Verification items for the finished model (mm, model axes). Face numbers are marked on the shaded views. A direction names the side the tool comes from. Coordinates: 2 decimals unless noted, no trailing zeros. Write each loop counter-clockwise with the first axis right and the second up, starting at its lowest first coordinate (ties: lowest second). Pieces come first, ordered by that corner, then holes. Notation, with made-up numbers: M 20.25,8.25 L 42.25,8.25 A24 ccw 42.25,18.25 Z; hole C -22.5,-13.75 d3. An arc over 180 degrees is marked long. One line per item, written item: value.
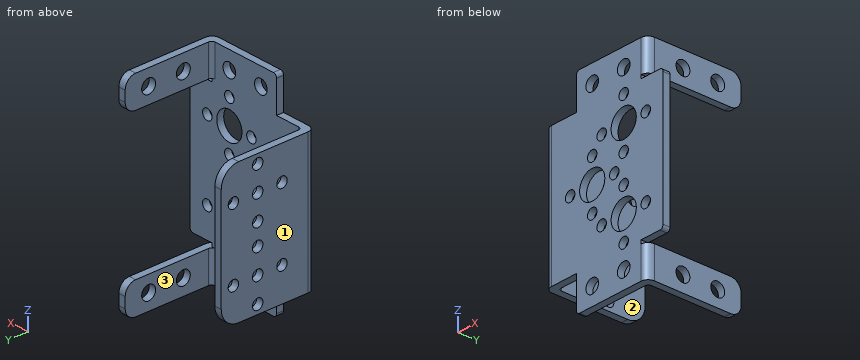
```python
from build123d import *

# Parameters (mm, degrees)
SKETCH1_W           = 35.49
SKETCH1_H           = 39
BOSS_EXTRUDE1_DEPTH = 2
SKETCH2_W           = 20.5
SKETCH2_H           = 10
BOSS_EXTRUDE2_DEPTH = 2
SKETCH3_W           = 39
SKETCH3_H           = 27
BOSS_EXTRUDE3_DEPTH = 2
SKETCH4_W           = 9
SKETCH4_H           = 27
BOSS_EXTRUDE4_DEPTH = 2
SKETCH5_R           = 4
SKETCH5_R_2         = 2
SKETCH5_R_3         = 1.5
CUT_EXTRUDE1_DEPTH  = 2
SKETCH6_R           = 2
CUT_EXTRUDE2_DEPTH  = 2
SKETCH7_R           = 1.5
CUT_EXTRUDE3_DEPTH  = 2
FILLET1_R           = 2
FILLET2_R           = 1
FILLET3_R           = 3
FILLET4_R           = 5


with BuildPart() as part:
    # Sketch1 → Boss-Extrude1 (new body)
    with BuildSketch(Plane(origin=(0, 0, 0), x_dir=(1, 0, 0), z_dir=(0, 1, 0))):
        Rectangle(SKETCH1_W, SKETCH1_H)
    extrude(amount=BOSS_EXTRUDE1_DEPTH)

    # Sketch2 → Boss-Extrude2 (add)
    with BuildSketch(Plane(origin=(0, 2, 0), x_dir=(1, 0, 0), z_dir=(0, 1, 0))):
        with Locations((0.505, 24.5)):
            Rectangle(SKETCH2_W, SKETCH2_H)
        with Locations((0.505, -24.5)):
            Rectangle(SKETCH2_W, SKETCH2_H)
    extrude(amount=-BOSS_EXTRUDE2_DEPTH)

    # Sketch3 → Boss-Extrude3 (add)
    with BuildSketch(Plane.ZY.offset(17.745)):
        with Locations((0, 13.5)):
            Rectangle(SKETCH3_W, SKETCH3_H)
    extrude(amount=BOSS_EXTRUDE3_DEPTH)

    # Sketch4 → Boss-Extrude4 (add)
    with BuildSketch(Plane(origin=(10.755, 0, 0), x_dir=(0, 0, -1), z_dir=(1, 0, 0))):
        with Locations((-25, 13.5)):
            Rectangle(SKETCH4_W, SKETCH4_H)
        with Locations((25, 13.5)):
            Rectangle(SKETCH4_W, SKETCH4_H)
    extrude(amount=BOSS_EXTRUDE4_DEPTH)

    # Sketch5 → Cut-Extrude1 (cut)
    with BuildSketch(Plane(origin=(0, 2, 0), x_dir=(1, 0, 0), z_dir=(0, 1, 0))):
        with Locations((-4.755, 0)):
            Circle(SKETCH5_R)
        with Locations((5.245, 11)):
            Circle(SKETCH5_R)
        with Locations((5.245, -11)):
            Circle(SKETCH5_R)
        with Locations((-4.755, -24.5)):
            Circle(SKETCH5_R_2)
        with Locations((5.245, -24.5)):
            Circle(SKETCH5_R_2)
        with Locations((5.245, 24.5)):
            Circle(SKETCH5_R_2)
        with Locations((5.245, 18)):
            Circle(SKETCH5_R_3)
        with Locations((12.245, 11)):
            Circle(SKETCH5_R_3)
        with Locations((5.245, 4)):
            Circle(SKETCH5_R_3)
        with Locations((-1.755, 11)):
            Circle(SKETCH5_R_3)
        with Locations((-4.755, 7)):
            Circle(SKETCH5_R_3)
        with Locations((2.245, 0)):
            Circle(SKETCH5_R_3)
        with Locations((-4.755, -7)):
            Circle(SKETCH5_R_3)
        with Locations((-11.755, 0)):
            Circle(SKETCH5_R_3)
        with Locations((5.245, -4)):
            Circle(SKETCH5_R_3)
        with Locations((12.245, -11)):
            Circle(SKETCH5_R_3)
        with Locations((5.245, -18)):
            Circle(SKETCH5_R_3)
        with Locations((-1.755, -11)):
            Circle(SKETCH5_R_3)
        with Locations((-4.755, 24.5)):
            Circle(SKETCH5_R_2)
    extrude(amount=-CUT_EXTRUDE1_DEPTH, mode=Mode.SUBTRACT)

    # Sketch6 → Cut-Extrude2 (cut)
    with BuildSketch(Plane(origin=(12.755, 0, 0), x_dir=(0, 0, -1), z_dir=(1, 0, 0))):
        with Locations((-25, 20.25)):
            Circle(SKETCH6_R)
        with Locations((-25, 10.25)):
            Circle(SKETCH6_R)
        with Locations((25, 20.25)):
            Circle(SKETCH6_R)
        with Locations((25, 10.25)):
            Circle(SKETCH6_R)
    extrude(amount=-CUT_EXTRUDE2_DEPTH, mode=Mode.SUBTRACT)

    # Sketch7 → Cut-Extrude3 (cut)
    with BuildSketch(Plane(origin=(-17.745, 0, 0), x_dir=(0, 0, -1), z_dir=(1, 0, 0))):
        with Locations((-10, 16.5)):
            Circle(SKETCH7_R)
        with Locations((-10, 23.5)):
            Circle(SKETCH7_R)
        with Locations((-3, 16.5)):
            Circle(SKETCH7_R)
        with Locations((-10, 9.5)):
            Circle(SKETCH7_R)
        with Locations((-17, 16.5)):
            Circle(SKETCH7_R)
        with Locations((10, 16.5)):
            Circle(SKETCH7_R)
        with Locations((10, 23.5)):
            Circle(SKETCH7_R)
        with Locations((17, 16.5)):
            Circle(SKETCH7_R)
        with Locations((10, 9.5)):
            Circle(SKETCH7_R)
        with Locations((3, 16.5)):
            Circle(SKETCH7_R)
    extrude(amount=-CUT_EXTRUDE3_DEPTH, mode=Mode.SUBTRACT)

    # Fillet1
    fillet1_edges = [part.edges().sort_by_distance(p)[0] for p in [
        (-19.745, 0, 0),
        (12.755, 0, -25),
        (12.755, 0, 25),
    ]]
    fillet(fillet1_edges, radius=FILLET1_R)

    # Fillet2
    fillet2_edges = [part.edges().sort_by_distance(p)[0] for p in [
        (-17.745, 2, 0),
        (10.755, 2, -25),
        (10.755, 2, 25),
        (-9.745, 1, -29.5),
        (17.745, 1, -19.5),
        (17.745, 1, 19.5),
        (-9.745, 1, 29.5),
    ]]
    fillet(fillet2_edges, radius=FILLET2_R)

    # Fillet3
    fillet3_edges = [part.edges().sort_by_distance(p)[0] for p in [
        (11.755, 27, 29.5),
        (11.755, 27, 20.5),
        (11.755, 27, -29.5),
        (11.755, 27, -20.5),
    ]]
    fillet(fillet3_edges, radius=FILLET3_R)

    # Fillet4
    fillet4_edges = [part.edges().sort_by_distance(p)[0] for p in [
        (-18.745, 27, -19.5),
        (-18.745, 27, 19.5),
    ]]
    fillet(fillet4_edges, radius=FILLET4_R)


solid = part.part
```
Item 1: Cross-section at D-D, the plane y = 19. Enter the section's corners in (x, z) (3 decimals).
The answers:
outline: M -19.745,-19.5 L -17.745,-19.5 L -17.745,19.5 L -19.745,19.5 Z; M 10.755,-29.5 L 12.755,-29.5 L 12.755,-26.561 L 10.755,-26.561 Z; M 10.755,-23.439 L 12.755,-23.439 L 12.755,-20.5 L 10.755,-20.5 Z; M 10.755,20.5 L 12.755,20.5 L 12.755,23.439 L 10.755,23.439 Z; M 10.755,26.561 L 12.755,26.561 L 12.755,29.5 L 10.755,29.5 Z
Item 2: Access from +Z, -Z, +X, -X, +Y, -Y to the whole of each face (thin tool, end or side, straight path). Record for the marked faces 1, 2 and 3.
The answers:
face 1: +Z, -Z, -X, +Y, -Y
face 2: +Z, -Z, +X, +Y
face 3: +Z, -Z, -X, +Y
Item 3: Cross-section at B-B, the plane y = 13. Enter the section's corners in (x, z) (3 decimals), and give its area (3 significant figures).
The answers:
outline: M -19.745,-19.5 L -17.745,-19.5 L -17.745,19.5 L -19.745,19.5 Z; M 10.755,-29.5 L 12.755,-29.5 L 12.755,-20.5 L 10.755,-20.5 Z; M 10.755,20.5 L 12.755,20.5 L 12.755,29.5 L 10.755,29.5 Z
area: 114 mm²
Item 4: Go/stop test with flat-tipped pins: P1, Ø1.6, axis at x = 13.5, y = 1, coming from the +Z side; P2, Ø8, axis at x = -14, y = 13.5, coming from the -Z side; P3, Ø4, axis at y = 15, z = 9, coming from the +X side (3 decimals); P4, Ø2.5, axis at x = -4.755, z = -7, coming from the -Y side. Record where each tip stops, or that it passes through.
The answers:
P1: stops at z = 19.5
P2: stops at z = -19.5
P3: stops at x = -17.745
P4: passes through
Item 5: Cross-section at A-A, the plane x = 8. Enter the section's corners in (y, z).
The answers:
outline: M 0,-29.5 L 2,-29.5 L 2,-13.9 L 0,-13.9 Z; M 0,-8.1 L 2,-8.1 L 2,8.1 L 0,8.1 Z; M 0,13.9 L 2,13.9 L 2,29.5 L 0,29.5 Z
Item 6: Scan lines: line 1 (Z direction, x = 12, y = 22.75); line 2 (X direction, y = 0.85, z = -24.5) (3 decimals); line 3 (X direction, y = 8, z = 0.5) (3 decimals). Record each from-to range of solid material in increasing order.
The answers:
line 1: z = -29.5 to -20.5, 20.5 to 29.5
line 2: x = -9.745 to -6.755, -2.755 to 3.245, 7.245 to 12.391
line 3: x = -19.745 to -17.745
Item 7: Cross-section at C-C, the plane z = 24.5. Enter the section's corners in (x, y) (1 decimal), and give its area (3 significant figures).
The answers:
outline: M -9.7,0 L -6.8,0 L -6.8,2 L -9.7,2 Z; M -2.8,0 L 3.2,0 L 3.2,2 L -2.8,2 Z; M 7.2,0 L 10.8,0 A2 ccw 12.8,2 L 12.8,8.3 L 10.8,8.3 L 10.8,3 A1 cw 9.8,2 L 7.2,2 Z; M 10.8,12.2 L 12.8,12.2 L 12.8,18.3 L 10.8,18.3 Z; M 10.8,22.2 L 12.8,22.2 L 12.8,27 L 10.8,27 Z
area: 62.9 mm²
